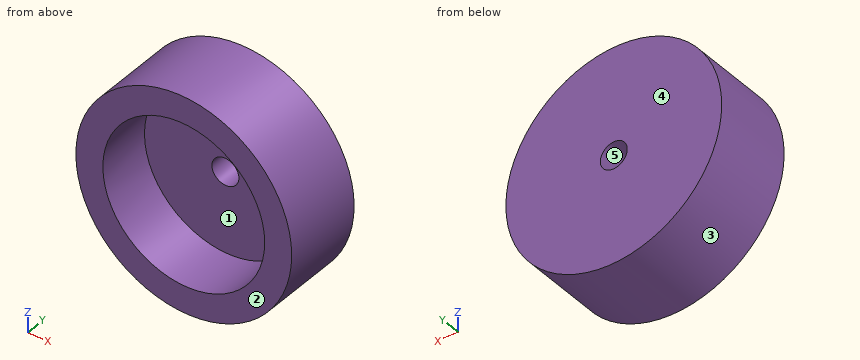
```python
from build123d import *

# Parameters (mm, degrees)
F0_R     = 50.8
F1_DEPTH = 38.1
F2_T     = -12.7
F3_R     = 6.35
F4_DEPTH = 38.101


with BuildPart() as f1:
    # F0 (on Front) → F1 (new body)
    with BuildSketch(Plane.XZ):
        Circle(F0_R)
    extrude(amount=-F1_DEPTH)

    # F2
    f2_openings = [f1.faces().sort_by_distance(p)[0] for p in [
        (0, 0, 0),
    ]]
    offset(amount=F2_T, openings=f2_openings)

    # F3 (on Front) → F4 (cut, through all)
    with BuildSketch(Plane.XZ):
        Circle(F3_R)
    extrude(amount=-F4_DEPTH, mode=Mode.SUBTRACT)


solid = f1.part
```
Source: CAD feature listing. Evaluate the final solid. Frame: model axes, mm. Face numbers are marked on the shaded views. A direction names the side the tool comes from. Round coordinates to 2 decimals unless told otherwise and drop trailing zeros. Loops run counter-clockwise (first coordinate to the right, second up) from the corner with the lowest first, then second, coordinate; pieces in that order, holes last. Notation, with made-up numbers: M 52.5,52 L 84.5,52 A17 cw 84.5,82 Z; hole C -14,28 d8. An arc over 180 degrees is marked long. Use a Markdown table: item, result. Add a question column.
1. Reachability of the marked faces 1 and 2 from +Z, -Z, +X, -X, +Y, -Y: full face, straight path, thin tool, end or side. Return the list, or none.
2. Section query D-D on y = 34. Return the cut outline in (x, z).
3. Section query B-B on z = 0. Return the cut outline in (x, y).
4. Mould query, pull axis Z, two halves, no side actions, for the marked faces 3, 4 and 5. Classes: pulls with the +Z half, pulls with the -Z half, needs draft (parallel to the pull), parting line crosses it, or undercut.
5. Section query C-C on z = -33. Return the cut outline in (x, y), then the cut area to 3 significant figures.
6. Contact query for flat-ended pins moving along their axis: P1, Ø3, axis at x = 24.5, z = -17, coming from the -Y side; P2, Ø5, axis at x = 1.5, y = 23.5, coming from the +Z side; P3, Ø1.5, axis at x = 3.5, y = 4.5, coming from the +Z side; P4, Ø10, axis at x = 0, z = 0, coming from the +Y side. Output: stop coordinate, or through.
7. Line query: line 1 (Z direction, x = 0, y = 34); line 2 (Z direction, x = 0, y = 15); line 3 (Y direction, x = 33, z = -6.5). Output: solid intervals per line, ascending.
8. Section query A-A on x = 0. Return the cut outline in (y, z).
Reported:
| question | item | result |
|---|---|---|
| 1 | face 1 | -Y |
| 1 | face 2 | +Z, -Z, +X, -X, -Y |
| 2 | outline | C 0,0 d101.6; hole C 0,0 d12.7 |
| 3 | outline | M -50.8,0 L -38.1,0 L -38.1,25.4 L -6.35,25.4 L -6.35,38.1 L -50.8,38.1 Z; M 6.35,25.4 L 38.1,25.4 L 38.1,0 L 50.8,0 L 50.8,38.1 L 6.35,38.1 Z |
| 4 | face 3 | parting line crosses it |
| 4 | face 4 | needs draft |
| 4 | face 5 | undercut |
| 5 | outline | M -38.62,0 L -19.04,0 L -19.04,25.4 L 19.04,25.4 L 19.04,0 L 38.62,0 L 38.62,38.1 L -38.62,38.1 Z |
| 5 | area | 1,980 mm² |
| 6 | P1 | stops at y = 25.4 |
| 6 | P2 | stops at z = 50.8 |
| 6 | P3 | stops at z = 50.73 |
| 6 | P4 | passes through |
| 7 | line 1 | z = -50.8 to -6.35, 6.35 to 50.8 |
| 7 | line 2 | z = -50.8 to -38.1, 38.1 to 50.8 |
| 7 | line 3 | y = 25.4 to 38.1 |
| 8 | outline | M 0,-50.8 L 38.1,-50.8 L 38.1,-6.35 L 25.4,-6.35 L 25.4,-38.1 L 0,-38.1 Z; M 0,38.1 L 25.4,38.1 L 25.4,6.35 L 38.1,6.35 L 38.1,50.8 L 0,50.8 Z |
